```python
from build123d import *

# Parameters (mm, degrees)
SKETCH_W     = 41
SKETCH_H     = 36
PAD_DEPTH    = 2
SKETCH001_W  = 37.3
SKETCH001_H  = 32.3
PAD001_DEPTH = 4
SKETCH002_W  = 34
SKETCH002_H  = 29
POCKET_DEPTH = 4
FILLET_R     = 1
FILLET001_R  = 1


with BuildPart() as part:
    # Sketch → Pad (new body)
    with BuildSketch(Plane.XY):
        Rectangle(SKETCH_W, SKETCH_H)
    extrude(amount=PAD_DEPTH)

    # Sketch001 (on Face6 of Pad) → Pad001 (join)
    with BuildSketch(Plane.XY.offset(2)):
        Rectangle(SKETCH001_W, SKETCH001_H)
    extrude(amount=PAD001_DEPTH)

    # Sketch002 (on Face11 of Pad001) → Pocket (cut)
    with BuildSketch(Plane.XY.offset(6)):
        Rectangle(SKETCH002_W, SKETCH002_H)
    extrude(amount=-POCKET_DEPTH, mode=Mode.SUBTRACT)

    # Fillet
    fillet_edges = [part.edges().sort_by_distance(p)[0] for p in [
        (0, 16.15, 6),
        (18.65, 0, 6),
        (0, -16.15, 6),
        (-18.65, 0, 6),
    ]]
    fillet(fillet_edges, radius=FILLET_R)

    # Fillet001
    fillet001_edges = [part.edges().sort_by_distance(p)[0] for p in [
        (0, 18, 0),
        (20.5, 0, 0),
        (0, -18, 0),
        (-20.5, 0, 0),
    ]]
    fillet(fillet001_edges, radius=FILLET001_R)


solid = part.part
```
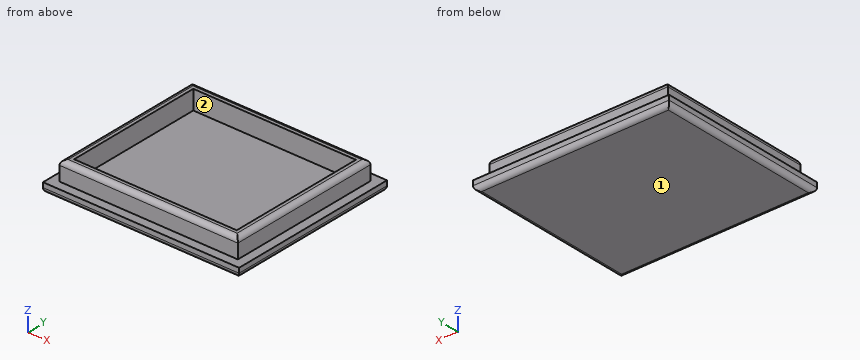
Geometry: final body of the model. Coordinates: model frame, mm. Face numbers are marked on the shaded views. Coordinates: 2 decimals unless noted, no trailing zeros. Order: outer loops, then holes, each group sorted by start corner. A loop starts at its lowest first (then second) coordinate and runs counter-clockwise, first axis right, second up. Notation, with made-up numbers: (34, 82) - (43, 82) arc R22 ccw to (43, 120) - close; hole circle Ø5 at (9.5, 82). An arc over 180 degrees is marked (long way). Write each question's results on one line, items separated by ' | '.
(1) Section query B-B, the plane z = 2.9. Return the cut outline in (x, y), plus the area to 3 significant figures.
Values found:
outline: (-18.65, -16.15) - (18.65, -16.15) - (18.65, 16.15) - (-18.65, 16.15) - close; hole (-17, -14.5) - (17, -14.5) - (17, 14.5) - (-17, 14.5) - close | area: 219 mm²
(2) First-contact query: pin 1 Ø3 at (y, z) = (-0.5, 4.5) entering from -X; pin 2 Ø0.9 at (x, z) = (4, 3) entering from -Y; pin 3 Ø1.5 at (x, z) = (10, 3) entering from +Y. Flat tips, straight axial feed; report the tip coordinate or a pass-through.
Values found:
pin 1: stops at x = -18.65 | pin 2: stops at y = -16.15 | pin 3: stops at y = 16.15
(3) Section query A-A, the plane x = 0. Return the cut outline in (y, z), plus the area to 3 significant figures.
Values found:
outline: (-18, 1) arc R1 ccw to (-17, 0) - (17, 0) arc R1 ccw to (18, 1) - (18, 2) - (16.15, 2) - (16.15, 5) arc R1 ccw to (15.15, 6) - (14.5, 6) - (14.5, 2) - (-14.5, 2) - (-14.5, 6) - (-15.15, 6) arc R1 ccw to (-16.15, 5) - (-16.15, 2) - (-18, 2) - close | area: 84.3 mm²
(4) Line query: line 1 (X direction, y = 3, z = 3.9); line 2 (Y direction, x = -2.5, z = 2.65). Output: solid intervals per line, ascending. Write a range as [from, to].
Values found:
line 1: x = [-18.65, -17], [17, 18.65] | line 2: y = [-16.15, -14.5], [14.5, 16.15]
(5) Section query D-D, the plane z = 5.5. Return the cut outline in (x, y).
Values found:
outline: (-18.52, -16.02) - (18.52, -16.02) - (18.52, 16.02) - (-18.52, 16.02) - close; hole (-17, -14.5) - (17, -14.5) - (17, 14.5) - (-17, 14.5) - close
(6) Section query C-C, the plane y = -5.5. Return the cut outline in (x, z), plus the area to 3 significant figures.
Values found:
outline: (-20.5, 1) arc R1 ccw to (-19.5, 0) - (19.5, 0) arc R1 ccw to (20.5, 1) - (20.5, 2) - (18.65, 2) - (18.65, 5) arc R1 ccw to (17.65, 6) - (17, 6) - (17, 2) - (-17, 2) - (-17, 6) - (-17.65, 6) arc R1 ccw to (-18.65, 5) - (-18.65, 2) - (-20.5, 2) - close | area: 94.3 mm²
(7) Mould query, pull axis Y, two halves, no side actions, for the marked faces 1 and 2. Classes: +Y half, -Y half, draft (parallel to the pull), parting line (faces both ways), or undercut.
Values found:
face 1: draft | face 2: undercut
